Source: CAD feature listing. Evaluate the final solid. Frame: model axes, mm. Face numbers are marked on the shaded views. Round coordinates to 2 decimals unless told otherwise and drop trailing zeros. Loops run counter-clockwise (first coordinate to the right, second up) from the corner with the lowest first, then second, coordinate; pieces in that order, holes last.
Item 1: Section query C-C on x = -31.5. Return loops of the section in (y, z), then the cut area to 3 significant figures.
Item 2: Ray query, L1, parallel to Z at x = -28, y = -11; L2, parallel to Y at x = 0, z = 39; L3, parallel to Y at x = 0, z = -1. Return the intervals inside material, ascending.
Item 3: Section query D-D on y = 33. Return loops of the section in (x, z).
Item 4: First-contact query: P1, Ø5, axis at x = 23, z = 6.5, coming from the +Y side; P2, Ø5, axis at x = 5.5, z = 13, coming from the -Y side; P3, Ø10, axis at y = -36, z = 73.5, coming from the +X side. Flat tips, straight axial feed; report the tip coordinate or a pass-through.
Item 5: Pull-direction query (Z, two-part tool) for the marked faces 1, 2 and 3; classes: released by +Z, released by -Z, zero draft, split by the parting line, or undercut.
Item 6: Section query A-A on x = 0. Return loops of the section in (y, z).
```python
from build123d import *

# Parameters (mm, degrees)
SKETCH1_R           = 48.137692039
SKETCH1_R_2         = 45.149668872
BOSS_EXTRUDE1_DEPTH = 83
SKETCH2_R           = 48.137692039
BOSS_EXTRUDE2_DEPTH = 3
BOSS_EXTRUDE3_START = 3
SKETCH3_R           = 48.137692039
BOSS_EXTRUDE3_DEPTH = 3
SKETCH4_R           = 20.853102152
CUT_EXTRUDE1_DEPTH  = 17


with BuildPart() as part:
    # Sketch1 → Boss-Extrude1 (new body)
    with BuildSketch(Plane.XY):
        Circle(SKETCH1_R)
        Circle(SKETCH1_R_2, mode=Mode.SUBTRACT)
    extrude(amount=BOSS_EXTRUDE1_DEPTH)

    # Sketch2 → Boss-Extrude2 (add)
    with BuildSketch(Plane.XY.offset(83)):
        Circle(SKETCH2_R)
    extrude(amount=BOSS_EXTRUDE2_DEPTH)

    # Sketch3 → Boss-Extrude3 (add)
    with BuildSketch(Plane(origin=(0, 0, 0), x_dir=(-1, 0, 0), z_dir=(0, 0, -1)).offset(BOSS_EXTRUDE3_START)):
        Circle(SKETCH3_R)
    extrude(amount=-BOSS_EXTRUDE3_DEPTH)

    # Sketch4 → Cut-Extrude1 (cut)
    with BuildSketch(Plane(origin=(0, 0, -3), x_dir=(-1, 0, 0), z_dir=(0, 0, -1))):
        Circle(SKETCH4_R)
    extrude(amount=-CUT_EXTRUDE1_DEPTH, mode=Mode.SUBTRACT)


solid = part.part
```
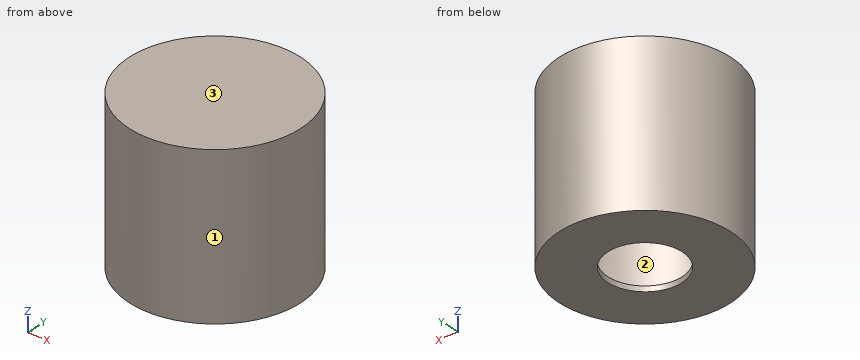
Data:
1. outline: (-36.4, -3) - (36.4, -3) - (36.4, 86) - (-36.4, 86) - close; hole (-32.35, 0) - (32.35, 0) - (32.35, 83) - (-32.35, 83) - close
1. area: 1,110 mm2
2. L1: z = -3 to 0, 83 to 86
2. L2: y = -48.14 to -45.15, 45.15 to 48.14
2. L3: y = -48.14 to -20.85, 20.85 to 48.14
3. outline: (-35.05, -3) - (35.05, -3) - (35.05, 86) - (-35.05, 86) - close; hole (-30.81, 0) - (30.81, 0) - (30.81, 83) - (-30.81, 83) - close
4. P1: stops at y = 43.55
4. P2: stops at y = -48.04
4. P3: stops at x = 36.83
5. face 1: zero draft
5. face 2: undercut
5. face 3: released by +Z
6. outline: (-48.14, -3) - (-20.85, -3) - (-20.85, 0) - (-45.15, 0) - (-45.15, 83) - (45.15, 83) - (45.15, 0) - (20.85, 0) - (20.85, -3) - (48.14, -3) - (48.14, 86) - (-48.14, 86) - close
